CAD build for the part. Positions are in the model's coordinates, mm. Face numbers are marked on the shaded views. Coordinates: 2 decimals unless noted, no trailing zeros. Loops run counter-clockwise (first coordinate to the right, second up) from the corner with the lowest first, then second, coordinate; pieces in that order, holes last. Notation, with made-up numbers: (-39, 5.25) -> (-12, 5.25) arc R9 cw to (-12, 11.25) -> close; hole circle Ø7 at (30, -14). An arc over 180 degrees is marked (long way). Write item = value, one per line. Start each with the question number.
(1) Pull direction Z, two halves, no side cores. Call the marked faces 1, 2, 3 and 4: +Z half, -Z half, draft (parallel to the pull), parting line (faces both ways), or undercut.
(2) Flat gauge pin, fed straight in: P1, Ø1, axis at x = -13.5, z = 16, coming from the +Y side. Where does the tip first touch, or does it go through?
(3) Band-saw the part on A-A (z = -8). Write the cut outline in (x, y).
(4) Band-saw the part on B-B (x = -10). Write the cut outline in (y, z), and give its area (3 significant figures).
(5) Drill centre lines: line 1 (Y direction, x = 1, z = 2); line 2 (Z direction, x = -23.5, y = -19.5); line 3 (X direction, y = -5.75, z = 24). Where is each one in solid material? Low to high. Write a range as from..to.
Autodesk Inventor part; units mm, degrees
ref_plane "YZ Plane" through (0, 0, 0) normal (1, 0, 0) x (0, 1, 0)
ref_plane "XZ Plane" through (0, 0, 0) normal (0, 1, 0) x (-1, 0, 0)
ref_plane "XY Plane" through (0, 0, 0) normal (0, 0, 1) x (1, 0, 0)
sketch "Sketch1" plane through (0, 0, 0) normal (0, 1, 0) x (-1, 0, 0)
  line L0 (50, 0) -> (-50, 0)
  line L1 (0, 50) -> (0, -50)
  line L2 (22, 27) -> (-22, 27)
  arc A0 (-22, 27) -> (-27, 22) centre (-22, 22) ccw
  line L3 (-27, 22) -> (-27, -22)
  arc A1 (-27, -22) -> (-22, -27) centre (-22, -22) ccw
  line L4 (-22, -27) -> (22, -27)
  arc A2 (22, -27) -> (27, -22) centre (22, -22) ccw
  line L5 (27, -22) -> (27, 22)
  arc A3 (27, 22) -> (22, 27) centre (22, 22) ccw
  point P0 (0, 0)
  dimension "d0" = 100
  dimension "d1" = 100
  dimension "core_outer_width" = 54
  dimension "core_outer_radius" = 5
extrude "Extrusion1" add sketch "Sketch1" against normal blind 25
sketch "Sketch2" plane through (0, 0, 0) normal (0, 1, 0) x (1, 0, 0)
  line L0 (-27, 22) -> (-27, -22) construction
  arc A0 (-27, -22) -> (-22, -27) centre (-22, -22) ccw construction
  line L1 (-22, -27) -> (22, -27) construction
  arc A1 (22, -27) -> (27, -22) centre (22, -22) ccw construction
  line L2 (27, -22) -> (27, 22) construction
  arc A2 (27, 22) -> (22, 27) centre (22, 22) ccw construction
  line L3 (22, 27) -> (-22, 27) construction
  arc A3 (-22, 27) -> (-27, 22) centre (-22, 22) ccw construction
  line L4 (22, -25.2) -> (-22, -25.2)
  arc A4 (-25.2, -22) -> (-22, -25.2) centre (-22, -22) ccw
  line L5 (-25.2, -22) -> (-25.2, 22)
  arc A5 (-22, 25.2) -> (-25.2, 22) centre (-22, 22) ccw
  line L6 (-22, 25.2) -> (22, 25.2)
  arc A6 (25.2, 22) -> (22, 25.2) centre (22, 22) ccw
  line L7 (25.2, 22) -> (25.2, -22)
  arc A7 (22, -25.2) -> (25.2, -22) centre (22, -22) ccw
  point P0 (0, 0)
  dimension "d6" = 1.8
extrude "Extrusion2" cut sketch "Sketch2" against normal blind 0.5
fillet "Fillet1" radius 0.2 16 edges at (-24.2627, -0.5, -24.2627) (0, -0.5, -25.2) (24.2627, -0.5, -24.2627) (25.2, -0.5, 0) (24.2627, -0.5, 24.2627) (0, -0.5, 25.2) (-24.2627, -0.5, 24.2627) (-25.2, -0.5, 0) (-24.2627, 0, -24.2627) (0, 0, -25.2) (24.2627, 0, -24.2627) (25.2, 0, 0) (24.2627, 0, 24.2627) (0, 0, 25.2) (-24.2627, 0, 24.2627) (-25.2, 0, 0)
equation "\"d6\" = -0.5 * core_inner_width + 0.5 * core_outer_width"
equation "\"core_inner_width\" = 50.4"
properties part number "core_dummy_1"
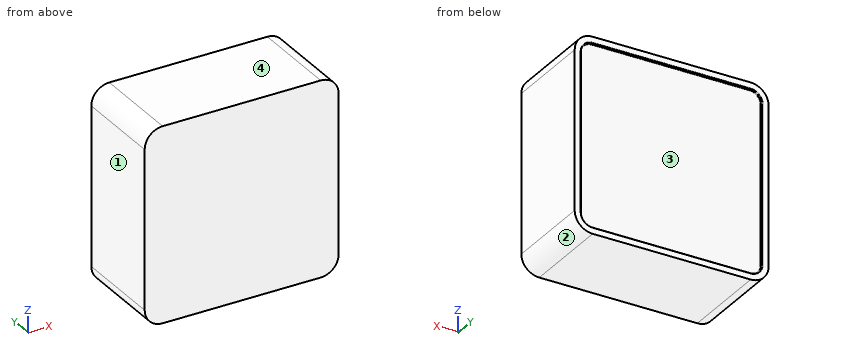
Findings below:
q1.face_1 = draft
q1.face_2 = -Z half
q1.face_3 = undercut
q1.face_4 = +Z half
q2.P1 = -0.5
q3.outline = (-27, -25) -> (27, -25) -> (27, 0) -> (25.4, 0) arc R0.2 ccw to (25.2, -0.2) -> (25.2, -0.3) arc R0.2 cw to (25, -0.5) -> (-25, -0.5) arc R0.2 cw to (-25.2, -0.3) -> (-25.2, -0.2) arc R0.2 ccw to (-25.4, 0) -> (-27, 0) -> close
q4.outline = (-25, -27) -> (0, -27) -> (0, -25.4) arc R0.2 ccw to (-0.2, -25.2) -> (-0.3, -25.2) arc R0.2 cw to (-0.5, -25) -> (-0.5, 25) arc R0.2 cw to (-0.3, 25.2) -> (-0.2, 25.2) arc R0.2 ccw to (0, 25.4) -> (0, 27) -> (-25, 27) -> close
q4.area = 1,320 mm²
q5.line_1 = -25..-0.5
q5.line_2 = -26.77..26.77
q5.line_3 = -26.58..26.58
